Build history of the part. All positions in model axes, mm. A direction names the side the tool comes from. Give positions to 0.01 mm unless a question says otherwise; leave off trailing zeros. Write each loop counter-clockwise with the first axis right and the second up, starting at its lowest first coordinate (ties: lowest second). Pieces come first, ordered by that corner, then holes.
from build123d import *

# Parameters (mm, degrees)
SCHIZZO1_W        = 94
SCHIZZO1_H        = 200
ESTRUSIONE1_DEPTH = 15
SCHIZZO2_W        = 18
SCHIZZO2_H        = 90
ESTRUSIONE2_DEPTH = 90
SCHIZZO3_R        = 7
ESTRUSIONE3_DEPTH = 90
SCHIZZO4_R        = 18
ESTRUSIONE4_DEPTH = 240.970831561
SCHIZZO5_R        = 20
ESTRUSIONE5_DEPTH = 20
SCHIZZO7_W        = 18
SCHIZZO7_H        = 90
ESTRUSIONE6_DEPTH = 40
SMUSSO1_SIZE      = 10


with BuildPart() as part:
    # Schizzo1 → Estrusione1 (new body)
    with BuildSketch(Plane(origin=(0, 0, 0), x_dir=(1, 0, 0), z_dir=(0, 1, 0))):
        with Locations((47, 100)):
            Rectangle(SCHIZZO1_W, SCHIZZO1_H)
    extrude(amount=ESTRUSIONE1_DEPTH)

    # Schizzo2 → Estrusione2 (add)
    with BuildSketch(Plane(origin=(0, 15, 0), x_dir=(1, 0, 0), z_dir=(0, 1, 0))):
        with Locations((72, 100)):
            Rectangle(SCHIZZO2_W, SCHIZZO2_H)
        with Locations((22, 100)):
            Rectangle(SCHIZZO2_W, SCHIZZO2_H)
    extrude(amount=ESTRUSIONE2_DEPTH)

    # Schizzo3 → Estrusione3 (cut)
    with BuildSketch(Plane(origin=(0, 15, 0), x_dir=(1, 0, 0), z_dir=(0, 1, 0))):
        with Locations(Location((47, 180, 0), (0, 0, 270))):
            Circle(SCHIZZO3_R)
        with Locations(Location((47, 20, 0), (0, 0, 270))):
            Circle(SCHIZZO3_R)
    extrude(amount=-ESTRUSIONE3_DEPTH, mode=Mode.SUBTRACT)

    # Schizzo4 → Estrusione4 (cut, through all)
    with BuildSketch(Plane(origin=(81, 0, 0), x_dir=(0, 0, -1), z_dir=(1, 0, 0))):
        with Locations((100, 70)):
            Circle(SCHIZZO4_R)
    extrude(amount=-ESTRUSIONE4_DEPTH, mode=Mode.SUBTRACT)

    # Schizzo5 → Estrusione5 (cut)
    with BuildSketch(Plane.ZY.offset(-13)):
        with Locations((-100, 70)):
            Circle(SCHIZZO5_R)
    extrude(amount=-ESTRUSIONE5_DEPTH, mode=Mode.SUBTRACT)

    # Schizzo7 → Estrusione6 (add)
    with BuildSketch(Plane(origin=(0, 105, 0), x_dir=(1, 0, 0), z_dir=(0, 1, 0))):
        with Locations((72, 100)):
            Rectangle(SCHIZZO7_W, SCHIZZO7_H)
    extrude(amount=ESTRUSIONE6_DEPTH)

    # Smusso1
    smusso1_edges = [part.edges().sort_by_distance(p)[0] for p in [
        (22, 105, -55),
        (22, 105, -145),
        (72, 145, -55),
        (72, 145, -145),
    ]]
    chamfer(smusso1_edges, length=SMUSSO1_SIZE)


solid = part.part
(1) Saw through at C-C, the plane z = -100. List the corners of the cut face in (x, y).
(2) Drop flat-ended pins along their axis: pin 1 (9 mm diameter, centred on x = 25.5, z = -90, fed in from +Y); pin 2 (6 mm diameter, centred on x = 81.5, z = -48, fed in from +Y); pin 3 (20 mm diameter, centred on x = 26, y = 70.5, fed in from +Z). Give the stop position or say it passes through.
(3) Saw through at D-D, the plane x = 27. List the corners of the cut face in (y, z).
(4) Probe line 1 (Y direction, x = 20.5, z = -100); line 2 (X direction, y = 7, z = -20); line 3 (Y direction, x = 21.5, z = -32.5). List the from-to ranges inside material, lowest first.
(5) Saw through at B-B, the plane y = 70. List the corners of the cut face in (x, z).
(6) Saw through at A-A, the plane x = 47. List the corners of the cut face in (y, z), plus the area to 3 significant figures.
(7) 3-axis set-ups, long thin cutter, end or side, ignore diameter. For faces 1 (the face through (22, 54, -145)), 2 (the face through (72, 74, -55)), 3 (the face through (22, 58, -116)): which of +Z, -Z, +X, -X, +Y, -Y reach the whole face in a straight line?
(8) Mould opens along X. For faces 4 (the face through (49.103, 7.605, -173.323)), 5 (the face through (22, 100, -140)), 6 (the face through (0, 7, -99)) say: +X half, -X half, draft (parallel to the pull), parting line (faces both ways), or undercut.
Computed values:
1. outline: (0, 0) - (94, 0) - (94, 15) - (81, 15) - (81, 52) - (63, 52) - (63, 15) - (31, 15) - (31, 50) - (13, 50) - (13, 15) - (0, 15) - close; (13, 90) - (31, 90) - (31, 105) - (13, 105) - close; (63, 88) - (81, 88) - (81, 145) - (63, 145) - close
2. pin 1: stops at y = 105
2. pin 2: stops at y = 15
2. pin 3: stops at z = -55
3. outline: (0, -200) - (15, -200) - (15, -145) - (95, -145) - (105, -135) - (105, -65) - (95, -55) - (15, -55) - (15, 0) - (0, 0) - close; hole circle Ø40 at (70, -100)
4. line 1: y = 0 to 50, 90 to 105
4. line 2: x = 0 to 40, 54 to 94
4. line 3: y = 0 to 15
5. outline: (13, -145) - (31, -145) - (31, -120) - (13, -120) - close; (13, -80) - (31, -80) - (31, -55) - (13, -55) - close; (63, -145) - (81, -145) - (81, -118) - (63, -118) - close; (63, -82) - (81, -82) - (81, -55) - (63, -55) - close
6. outline: (0, -200) - (15, -200) - (15, -187) - (0, -187) - close; (0, -173) - (15, -173) - (15, -27) - (0, -27) - close; (0, -13) - (15, -13) - (15, 0) - (0, 0) - close
6. area: 2,580 mm2
7. face 1: -Z, +X, -X, +Y
7. face 2: +Z, +X, -X, +Y
7. face 3: -X
8. face 4: undercut
8. face 5: draft
8. face 6: -X half
